Here's how the part is built. I have some questions about the finished solid (model axes, mm). A direction names the side the tool comes from. Round coordinates to 2 decimals unless told otherwise and drop trailing zeros. Loops run counter-clockwise (first coordinate to the right, second up) from the corner with the lowest first, then second, coordinate; pieces in that order, holes last. Notation, with made-up numbers: M 77.5,48 L 106.5,48 A29 cw 106.5,80 Z; hole C 83,17.25 d9. An arc over 180 degrees is marked long. Answer as a JSON object with one key per item and string values.
from build123d import *

# Parameters (mm, degrees)
SKETCH1_W           = 46.35
SKETCH1_H           = 27.35
BOSS_EXTRUDE1_DEPTH = 14
BOSS_EXTRUDE2_DEPTH = 3.175


with BuildPart() as part:
    # Sketch1 → Boss-Extrude1 (new body)
    with BuildSketch(Plane.XY):
        Rectangle(SKETCH1_W, SKETCH1_H)
    extrude(amount=BOSS_EXTRUDE1_DEPTH)

    # Sketch2 → Boss-Extrude2 (add)
    with BuildSketch(Plane.XY):
        with BuildLine():
            Line((23.175, 6.604134349), (30.60317409, 4.6137611))
            ThreePointArc((30.60317409, 4.6137611), (31.504475179, 3.264868697), (30.284766137, 2.195212576))
            Line((30.284766137, 2.195212576), (25.885652609, 2.195212576))
            ThreePointArc((25.885652609, 2.195212576), (23.690440034, 0), (25.885652609, -2.195212576))
            Line((25.885652609, -2.195212576), (30.284766137, -2.195212576))
            ThreePointArc((30.284766137, -2.195212576), (31.504475179, -3.264868697), (30.60317409, -4.6137611))
            Line((30.60317409, -4.6137611), (23.175, -6.604134349))
            Line((23.175, -6.604134349), (23.175, 6.604134349))
        make_face()
    boss_extrude2 = extrude(amount=BOSS_EXTRUDE2_DEPTH)

    # Mirror1: Boss-Extrude2 across plane
    add(boss_extrude2.mirror(Plane(origin=(0, 0, 0), x_dir=(0, 0, 1), z_dir=(1, 0, 0))))


solid = part.part
Item 1: Please list where these lines run through material, in increasing order: probe 1 along X at (y, z) = (-11.75, 6.75) (3 decimals); probe 2 along Y at (x, z) = (28, 2.75); probe 3 along Y at (x, z) = (29, 2). Write a range as from..to.
Resolved:
{"probe 1": "-23.175..23.175", "probe 2": "-5.31..-2.2, 2.2..5.31", "probe 3": "-5.04..-2.2, 2.2..5.04"}
Item 2: I want a section at D-D, the plane y = -11. Please give me the cut outline in (x, z) (3 decimals).
Resolved:
{"outline": "M -23.175,0 L 23.175,0 L 23.175,14 L -23.175,14 Z"}
Item 3: If we mould it in two halves opening along Y, with no side actions, what happens to faces 1 (the face through (-28, 2.195, 2)), 2 (the face through (0, 0, 0)), 3 (the face through (-26.837, 5.623, 1.565))? For each: pulls with the +Y half, pulls with the -Y half, needs draft (parallel to the pull), parting line crosses it, or undercut.
Resolved:
{"face 1": "undercut", "face 2": "needs draft", "face 3": "pulls with the +Y half"}
Item 4: I want a section at A-A, the plane x = -27.5. Please give me the cut outline in (y, z) (3 decimals).
Resolved:
{"outline": "M -5.445,0 L -2.195,0 L -2.195,3.175 L -5.445,3.175 Z; M 2.195,0 L 5.445,0 L 5.445,3.175 L 2.195,3.175 Z"}
Item 5: On a 3-axis mill with a long thin cutter (end or side, diameter ignored), from which of +Z, -Z, +X, -X, +Y, -Y can I reach the whole of each face in a straight line? I mean faces 4 (the face through (-26.941, -5.595, 1.565)), 5 (the face through (26, -3, 3.175)), 6 (the face through (-28, -2.195, 2)), 7 (the face through (28, -2.195, 2)), 8 (the face through (26.941, -5.595, 1.565)). Say none if no direction works.
Resolved:
{"face 4": "+Z, -Z, -X, -Y", "face 5": "+Z, +X, +Y, -Y", "face 6": "+Z, -Z, -X", "face 7": "+Z, -Z, +X", "face 8": "+Z, -Z, +X, -Y"}
Item 6: I want a section at B-B, the plane y = 0. Please give me the cut outline in (x, z) (3 decimals).
Resolved:
{"outline": "M -23.69,0 L 23.69,0 L 23.69,3.175 L 23.175,3.175 L 23.175,14 L -23.175,14 L -23.175,3.175 L -23.69,3.175 Z"}
Item 7: I want a section at C-C, the plane z = 13.25. Please give me the cut outline in (x, y) (3 decimals), then the cut area to 3 significant figures.
Resolved:
{"outline": "M -23.175,-13.675 L 23.175,-13.675 L 23.175,13.675 L -23.175,13.675 Z", "area": "1,270 mm²"}
Item 8: I'm going to push flat-ended pins straight in: pin 1 Ø4 at (x, y) = (26.5, 2.5) entering from +Z (3 decimals); pin 2 Ø1 at (x, z) = (29, 2) entering from +Y; pin 3 Ø3.5 at (x, z) = (-27, 2) entering from +Y. Where does each tip first touch, or does it pass through?
Resolved:
{"pin 1": "z = 3.175", "pin 2": "y = 5.18", "pin 3": "y = 6.05"}
